from build123d import *

# Parameters (mm, degrees)
SKETCH2_R            = 3
BOSS_EXTRUDE1_DEPTH  = 20
FILLET1_R            = 6
FILLET2_R            = 2
FILLET4_R            = 5
SKETCH3_W            = 30
SKETCH3_H            = 12
SKETCH3_R            = 3.25
BOSS_EXTRUDE2_DEPTH  = 10
FILLET3_R            = 6
FILLET3_OF_MIRROR1_R = 6
BOSS_EXTRUDE3_DEPTH  = 40


# Some blends are built 0.0001 mm under size
with BuildPart() as part:
    # Sketch2 → Boss-Extrude1 (new, symmetric)
    with BuildSketch(Plane.XY):
        with BuildLine():
            Line((-6, 6), (6, 6))
            Line((6, 6), (6, -10.886905517))
            Line((6, -10.886905517), (3, -17.320426279))
            Line((3, -17.320426279), (6, -23.75394704))
            ThreePointArc((6, -23.75394704), (12.097077324, -21.305180596), (17.324116139, -17.324116139))
            Line((17.324116139, -17.324116139), (22.980970389, -22.980970389))
            ThreePointArc((22.980970389, -22.980970389), (19.899357283, -25.695633476), (16.5, -28))
            Line((16.5, -28), (6, -28))
            Line((6, -28), (-6, -16))
            Line((-6, -16), (-6, 6))
        make_face()
        Circle(SKETCH2_R, mode=Mode.SUBTRACT)
    extrude(amount=BOSS_EXTRUDE1_DEPTH, both=True)

    # Fillet1
    fillet1_edges = [part.edges().sort_by_distance(p)[0] for p in [
        (6, 6, 0),
        (-6, 6, 0),
    ]]
    fillet(fillet1_edges, radius=FILLET1_R - 0.0001)  # a hair under: the kernel refuses the full size

    # Fillet2
    fillet2_edges = [part.edges().sort_by_distance(p)[0] for p in [
        (17.324116139, -17.324116139, 0),
        (22.980970389, -22.980970389, 0),
        (16.5, -28, 0),
        (6, -28, 0),
        (-6, -16, 0),
    ]]
    fillet(fillet2_edges, radius=FILLET2_R)

    # Fillet4
    fillet4_edges = [part.edges().sort_by_distance(p)[0] for p in [
        (6, -10.886905517, 0),
        (3, -17.320426279, 0),
        (6, -23.75394704, 0),
    ]]
    fillet(fillet4_edges, radius=FILLET4_R)

    # Sketch3 → Boss-Extrude2 (add)
    with BuildSketch(Plane.XY.offset(20)):
        with Locations((-21, -8)):
            Rectangle(SKETCH3_W, SKETCH3_H)
        with Locations((-30, -8)):
            Circle(SKETCH3_R, mode=Mode.SUBTRACT)
    boss_extrude2 = extrude(amount=-BOSS_EXTRUDE2_DEPTH)

    # Fillet3
    # the kernel refuses this fillet: 6 mm, written as the material it adds along each edge
    with BuildSketch(Plane(origin=(-6, -14, 20), x_dir=(0.16798992441845362, -0.9857887122978647, 0), z_dir=(0, 0, -1))) as fillet3_piece_1:
        with BuildLine():
            CenterArc((5.179174836, 5.324294957), FILLET3_R, 189.670969531, 52.875183342)
            Line((-0.735557438, 4.316355411), (-1.327030665, 4.215561456))
            Line((-1.327030665, 4.215561456), (-0.591473227, -0.100793955))
            Line((-0.591473227, -0.100793955), (0.100793955, -0.591473227))
            ThreePointArc((0.100793955, -0.591473227), (1.255717271, -0.394660789), (2.136350707, -0.532429496))
            Line((2.136350707, -0.532429496), (2.412971083, 0))
        make_face()
    extrude(amount=10)
    with BuildSketch(Plane(origin=(-6, -2, 20), x_dir=(0.08546746952976336, 0.9963409615448815, 0), z_dir=(0, 0, -1))) as fillet3_piece_2:
        with BuildLine():
            CenterArc((5.523894047, -5.807099434), FILLET3_R, 104.567976289, 70.529116987)
            Line((-0.454151722, -5.294294617), (-1.051956299, -5.243014135))
            Line((-1.051956299, -5.243014135), (-0.597804577, 0.051280482))
            Line((-0.597804577, 0.051280482), (0.051280482, 0.597804577))
            ThreePointArc((0.051280482, 0.597804577), (2.044062039, 0.426861091), (3.863806292, 0.580709943))
            Line((3.863806292, 0.580709943), (4.014723361, 0))
        make_face()
    extrude(amount=10)
    # the kernel refuses this fillet: 6 mm, written as the material it takes off along each edge
    with BuildSketch(Plane(origin=(-36, -14, 35), x_dir=(0, 1, 0), z_dir=(0, 0, -1)), Plane(origin=(-36, -2, 35), x_dir=(1, 0, 0), z_dir=(0, 0, -1))) as fillet3_2_piece_1:
        with BuildLine():
            CenterArc((FILLET3_R, FILLET3_R), FILLET3_R, 180, 90)
            Line((0, FILLET3_R), (0, 0))
            Line((0, 0), (FILLET3_R, 0))
        make_face()
    extrude(amount=40, mode=Mode.SUBTRACT)

    # Mirror1: Boss-Extrude2 across plane
    add(boss_extrude2.mirror(Plane.XY))

    # Fillet3 of Mirror1
    # the kernel refuses this fillet: 6 mm, written as the material it adds along each edge
    with BuildSketch(Plane(origin=(-6, -14, -20), x_dir=(0.16798992441845362, -0.9857887122978647, 0), z_dir=(0, 0, 1))) as fillet3_of_mirror1_piece_1:
        with BuildLine():
            CenterArc((5.179174836, -5.324294957), FILLET3_OF_MIRROR1_R, 117.453847127, 52.875183342)
            Line((-0.735557438, -4.316355411), (-1.327030665, -4.215561456))
            Line((-1.327030665, -4.215561456), (-0.591473227, 0.100793955))
            Line((-0.591473227, 0.100793955), (0.100793955, 0.591473227))
            ThreePointArc((0.100793955, 0.591473227), (1.255717271, 0.394660789), (2.136350707, 0.532429496))
            Line((2.136350707, 0.532429496), (2.412971083, 0))
        make_face()
    extrude(amount=10)
    with BuildSketch(Plane(origin=(-6, -2, -20), x_dir=(0.08546746952976336, 0.9963409615448815, 0), z_dir=(0, 0, 1))) as fillet3_of_mirror1_piece_2:
        with BuildLine():
            CenterArc((5.523894047, 5.807099434), FILLET3_OF_MIRROR1_R, 184.902906724, 70.529116987)
            Line((-0.454151722, 5.294294617), (-1.051956299, 5.243014135))
            Line((-1.051956299, 5.243014135), (-0.597804577, -0.051280482))
            Line((-0.597804577, -0.051280482), (0.051280482, -0.597804577))
            ThreePointArc((0.051280482, -0.597804577), (2.044062039, -0.426861091), (3.863806292, -0.580709943))
            Line((3.863806292, -0.580709943), (4.014723361, 0))
        make_face()
    extrude(amount=10)
    # the kernel refuses this fillet: 6 mm, written as the material it takes off along each edge
    with BuildSketch(Plane(origin=(-36, -14, -35), x_dir=(1, 0, 0), z_dir=(0, 0, 1)), Plane(origin=(-36, -2, -35), x_dir=(0, -1, 0), z_dir=(0, 0, 1))) as fillet3_of_mirror1_2_piece_1:
        with BuildLine():
            CenterArc((FILLET3_OF_MIRROR1_R, FILLET3_OF_MIRROR1_R), FILLET3_OF_MIRROR1_R, 180, 90)
            Line((0, FILLET3_OF_MIRROR1_R), (0, 0))
            Line((0, 0), (FILLET3_OF_MIRROR1_R, 0))
        make_face()
    extrude(amount=40, mode=Mode.SUBTRACT)

    # Sketch4 → Boss-Extrude3 (add)
    with BuildSketch(Plane(origin=(0, 0, -20), x_dir=(-1, 0, 0), z_dir=(0, 0, -1))):
        with BuildLine():
            Line((-2.4, 1.8), (2.4, 1.8))
            ThreePointArc((2.4, 1.8), (0, 3), (-2.4, 1.8))
        make_face()
    extrude(amount=-BOSS_EXTRUDE3_DEPTH)


solid = part.part
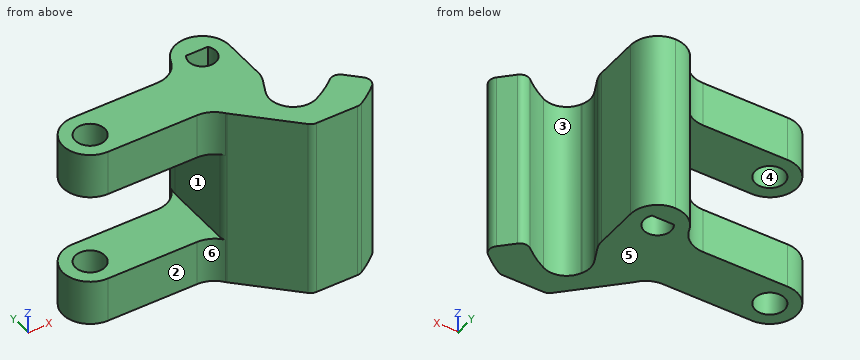
Could you check a few things on this model? Use its own coordinates, in mm. Face numbers are marked on the shaded views. A direction names the side the tool comes from. Round coordinates to 2 decimals unless told otherwise and drop trailing zeros. Write each loop counter-clockwise with the first axis right and the second up, starting at its lowest first coordinate (ties: lowest second). Pieces come first, ordered by that corner, then holes. Notation, with made-up numbers: (-6, 55) - (26, 55) arc R14 ccw to (26, 75) - close; hole circle Ø8 at (9, 22). An arc over 180 degrees is marked (long way). Put each result on its own line as item: value. Start each with the question number.
(1) For the marked faces 1, 2 and 3, which set-ups out of +Z, -Z, +X, -X, +Y, -Y let a thin tool reach every point of the face, with its end or its side?
(2) I need wall thicknesses on probe 1 along Y at (x, z) = (-30, -12); probe 2 along Z at (x, y) = (-29, -4.5); probe 3 along X at (y, z) = (-6, -4.5). Which ranges of each line are inside material? Lowest first, please.
(3) Thinking about a two-plate mould opening in Y: for the marked faces 4, 5 and 6, which applies, released by +Y, released by -Y, zero draft, split by the parting line, or undercut?
(4) Will these pins go through, and if not, where does the flat tip stop? pin 1 (6 mm diameter, centred on y = -10.5, z = 13.5, fed in from -X); pin 2 (1.5 mm diameter, centred on x = 14, z = -14, fed in from +Y); pin 3 (4.5 mm diameter, centred on y = -7, z = 4.5, fed in from -X); pin 4 (4 mm diameter, centred on x = 0.5, z = -5, fed in from -Y).
(5) I want a section at A-A, the plane z = 17. Give the number of separate pieces and of enclosed holes in the cut face, plus the area to 3 significant figures.
(6) I want a section at C-C, the plane y = -8. Please give me the cut outline in (x, z).
(7) I want a section at B-B, the plane x = -26. Please give me the cut outline in (y, z).
Here are the results:
1. face 1: -X, +Y, -Y
1. face 2: +Z, -Z, -X, -Y
1. face 3: +Z, -Z
2. probe 1: y = -14 to -11.25, -4.75 to -2
2. probe 2: z = -20 to -10, 10 to 20
2. probe 3: x = -6 to 6
3. face 4: undercut
3. face 5: zero draft
3. face 6: released by -Y
4. pin 1: stops at x = -36
4. pin 2: stops at y = -19.56
4. pin 3: stops at x = -6
4. pin 4: stops at y = -24.5
5. separate pieces: 1
5. enclosed holes: 2
5. area: 706 mm^2
6. outline: (-36, -20) - (-33.25, -20) - (-33.25, -10) - (-36, -10) - close; (-36, 10) - (-33.25, 10) - (-33.25, 20) - (-36, 20) - close; (-26.75, -20) - (6, -20) - (6, 20) - (-26.75, 20) - (-26.75, 10) - (-6, 10) - (-6, -10) - (-26.75, -10) - close
7. outline: (-14, -20) - (-2, -20) - (-2, -10) - (-14, -10) - close; (-14, 10) - (-2, 10) - (-2, 20) - (-14, 20) - close
